Verification items for the finished model (mm, model axes). A direction names the side the tool comes from. Round coordinates to 2 decimals unless told otherwise and drop trailing zeros. Write each loop counter-clockwise with the first axis right and the second up, starting at its lowest first coordinate (ties: lowest second). Pieces come first, ordered by that corner, then holes.
from build123d import *

# Parameters (mm, degrees)
SKETCH1_R           = 57.5
SKETCH1_R_2         = 1.89865
SKETCH1_R_3         = 1.9939
SKETCH1_R_4         = 8
BOSS_EXTRUDE1_DEPTH = 6.35
CUT_EXTRUDE1_DEPTH  = 82.564836173
SKETCH3_W           = 6.35
SKETCH3_H           = 80
CUT_EXTRUDE3_DEPTH  = 82.564836173
CUT_EXTRUDE5_DEPTH  = 82.564836173
CUT_EXTRUDE6_DEPTH  = 78.899883665


with BuildPart() as part:
    # Sketch1 → Boss-Extrude1 (new body)
    with BuildSketch(Plane.XY):
        Circle(SKETCH1_R)
        with Locations((45.315389352, 21.130913087)):
            Circle(SKETCH1_R_2, mode=Mode.SUBTRACT)
        with Locations((49.978847504, 1.454235937)):
            Circle(SKETCH1_R_3, mode=Mode.SUBTRACT)
        Circle(SKETCH1_R_4, mode=Mode.SUBTRACT)
        with Locations((46.467376211, -18.460307366)):
            Circle(SKETCH1_R_3, mode=Mode.SUBTRACT)
        with Locations((0, -16.5)):
            Circle(SKETCH1_R_3, mode=Mode.SUBTRACT)
        with Locations((0, -50)):
            Circle(SKETCH1_R_2, mode=Mode.SUBTRACT)
        with Locations((-16.5, 0)):
            Circle(SKETCH1_R_3, mode=Mode.SUBTRACT)
        with Locations((-11.66726189, -11.66726189)):
            Circle(SKETCH1_R_2, mode=Mode.SUBTRACT)
        with Locations((0, 16.5)):
            Circle(SKETCH1_R_3, mode=Mode.SUBTRACT)
        with Locations((-11.66726189, 11.66726189)):
            Circle(SKETCH1_R_2, mode=Mode.SUBTRACT)
        with Locations((11.66726189, 11.66726189)):
            Circle(SKETCH1_R_2, mode=Mode.SUBTRACT)
        with Locations((-35.355339059, -35.355339059)):
            Circle(SKETCH1_R_2, mode=Mode.SUBTRACT)
        with Locations((-50, 0)):
            Circle(SKETCH1_R_2, mode=Mode.SUBTRACT)
        with Locations((-35.355339059, 35.355339059)):
            Circle(SKETCH1_R_2, mode=Mode.SUBTRACT)
        with Locations((0, 50)):
            Circle(SKETCH1_R_2, mode=Mode.SUBTRACT)
        with Locations((35.355339059, -35.355339059)):
            Circle(SKETCH1_R_2, mode=Mode.SUBTRACT)
    extrude(amount=BOSS_EXTRUDE1_DEPTH)

    # Sketch2 → Cut-Extrude1 (cut, through all)
    with BuildSketch(Plane.XY):
        Polygon((12.5, -29.35), (41, -29.35), (41, 10.65), (44.5, 10.65), (44.5, 17), (41, 17), (41, 32), (21, 32), (21, 17), (17.5, 17), (17.5, 10.65), (21, 10.65), (21, 5.65), (12.5, 5.65), align=None)
    extrude(amount=CUT_EXTRUDE1_DEPTH, mode=Mode.SUBTRACT)

    # Sketch3 → Cut-Extrude3 (cut, through all)
    with BuildSketch(Plane(origin=(0, 0, 0), x_dir=(-1, 0, 0), z_dir=(0, 0, -1))):
        with Locations((-31, 32)):
            Rectangle(SKETCH3_W, SKETCH3_H)
    extrude(amount=-CUT_EXTRUDE3_DEPTH, mode=Mode.SUBTRACT)

    # Sketch4 → Cut-Extrude5 (cut, through all)
    with BuildSketch(Plane.XY):
        with BuildLine():
            Line((21, -36.500002949), (21, -5.372089924))
            Line((21, -5.372089924), (24.175, -5.411516926))
            Line((24.175, -5.411516926), (24.175, -57.5))
            Line((24.175, -57.5), (2.949e-06, -57.5))
            ThreePointArc((2.949e-06, -57.5), (14.849243269, -51.349243269), (21, -36.500002949))
        make_face()
        with BuildLine():
            Line((2.949e-06, 57.5), (24.175, 57.5))
            Line((24.175, 57.5), (24.175, 5.411516926))
            Line((24.175, 5.411516926), (21, 5.372089924))
            Line((21, 5.372089924), (21, 36.500002949))
            ThreePointArc((21, 36.500002949), (14.849243269, 51.349243269), (2.949e-06, 57.5))
        make_face()
    extrude(amount=CUT_EXTRUDE5_DEPTH, mode=Mode.SUBTRACT)


with BuildPart() as cut_extrude5_piece_1:
    # of the separate pieces the step leaves, piece 1, a body of its own (cut_extrude5_pieces_kept)
    add(part.part.solids().sort_by_distance((24.175, -52.171058787, 0))[0])


with BuildPart() as cut_extrude5_piece_2:
    # of the separate pieces the step leaves, piece 2, a body of its own (cut_extrude5_pieces_kept)
    add(part.part.solids().sort_by_distance((24.175, 52.171058787, 6.35))[0])

    # Sketch5 → Cut-Extrude6 (cut, through all)
    with BuildSketch(Plane.XY.offset(6.35)):
        with BuildLine():
            Line((24.175, 52.171058787), (24.175, 32))
            Line((24.175, 32), (27.825, 32))
            Line((27.825, 32), (27.825, 50.319175023))
            ThreePointArc((27.825, 50.319175023), (26.016482629, 51.277603607), (24.175, 52.171058787))
        make_face()
    extrude(amount=-CUT_EXTRUDE6_DEPTH, mode=Mode.SUBTRACT)


solid = cut_extrude5_piece_1.part
Q1. Sectioned sample at B-B (z = 1.75). Enter the section's corners in (x, y) (3 decimals), plus the area to 3 significant figures.
Recorded:
outline: (24.175, -52.171) arc R57.5 ccw to (34.175, 46.242) - (34.175, 32) - (41, 32) - (41, 17) - (44.5, 17) - (44.5, 10.65) - (41, 10.65) - (41, -29.35) - (24.175, -29.35) - close; hole circle Ø3.797 at (35.355, -35.355); hole circle Ø3.797 at (45.315, 21.131); hole circle Ø3.988 at (46.467, -18.46); hole circle Ø3.988 at (49.979, 1.454)
area: 1,220 mm2
Q2. Depth check by flat-ended pin: P1, Ø1, axis at x = 51, z = 4.5, coming from the +Y side; P2, Ø1, axis at x = 43, z = 1.5, coming from the -Y side; P3, Ø3, axis at y = 12.5, z = 4.5, coming from the -X side; P4, Ø3.5, axis at x = 46.47, y = -18.46, coming from the +Z side. Enter the tip coordinate at first touch or a pass-through.
Recorded:
P1: stops at y = 27.5
P2: stops at y = -38.73
P3: stops at x = 44.5
P4: passes through
Q3. Material ranges on line 1 along Y through (x, z) = (45, 1); line 2 along Y through (x, z) = (35.5, 3); line 3 along X through (y, z) = (-37, 1.75) (3 decimals), recorded low to high.
Recorded:
line 1: y = -35.79 to -19.81, -17.11 to 19.26, 23 to 35.79
line 2: y = -45.23 to -37.25, -33.46 to -29.35, 32 to 45.23
line 3: x = 24.175 to 34.407, 36.304 to 44.014
Q4. Sectioned sample at C-C (y = -12.5). Enter the section's corners in (x, z).
Recorded:
outline: (41, 0) - (56.12, 0) - (56.12, 6.35) - (41, 6.35) - close
Q5. Sectioned sample at A-A (x = 51). Enter the section's corners in (y, z), plus the area to 3 significant figures.
Recorded:
outline: (-26.56, 0) - (-0.26, 0) - (-0.26, 6.35) - (-26.56, 6.35) - close; (3.17, 0) - (26.56, 0) - (26.56, 6.35) - (3.17, 6.35) - close
area: 316 mm2
Q6. Tool access check on faces 1 (the flat face through (32, -29.35, 3)), 2 (the flat face through (43, -6, 0)). Record the directions out of +Z, -Z, +X, -X, +Y, -Y that give a thin tool (end or side, any length) a straight path to the whole face; none if there is none.
Recorded:
face 1: +Z, -Z, -X
face 2: -Z, +X, -X, +Y, -Y
Q7. Sectioned sample at D-D (x = 27). Enter the section's corners in (y, z), plus the area to 3 significant figures.
Recorded:
outline: (-50.77, 0) - (-29.35, 0) - (-29.35, 6.35) - (-50.77, 6.35) - close
area: 136 mm2
Q8. Release check for a two-part mould opening along X. For faces 3 (the cylindrical face through (44.475, -18.373, 3.131)), 4 (the flat face through (34.175, 39, 3)), 5 (the flat face through (43, -6, 6.35)) record: released by +X, released by -X, zero draft, split by the parting line, or undercut.
Recorded:
face 3: undercut
face 4: released by -X
face 5: zero draft
